from build123d import *

# Parameters (mm, degrees)
F0_R     = 3
F1_DEPTH = 15
F2_W     = 7
F2_H     = 5
F3_DEPTH = 10
F4_F1_R  = 2
F4_F2_R  = 2
F5_R     = 2


with BuildPart() as f1:
    # F0 (on Top) → F1 (new body)
    with BuildSketch(Plane.XY):
        with BuildLine():
            Line((-40.4142135624, -39), (-4.8904069139, -3.4761933515))
            ThreePointArc((-4.8904069139, -3.4761933515), (5.9789831367, -0.5017575617), (-4.2426406871, 4.2426406871))
            Line((-4.2426406871, 4.2426406871), (-42.4852813742, -34))
            Line((-42.4852813742, -34), (-104.8479702921, -34))
            Line((-104.8479702921, -34), (-87.5274622164, -44))
            Line((-87.5274622164, -44), (-90.4142135624, -39))
            Line((-90.4142135624, -39), (-40.4142135624, -39))
        make_face()
        Circle(F0_R, mode=Mode.SUBTRACT)
    extrude(amount=F1_DEPTH)

    # F2 (on face) → F3 (join)
    with BuildSketch(Plane(origin=(-4.2426406871, 4.2426406871, 0), x_dir=(-0.7071067812, -0.7071067812, 0), z_dir=(-0.7071067812, 0.7071067812, 0))):
        with Locations((36.5832611207, 7.5)):
            Rectangle(F2_W, F2_H)
    extrude(amount=F3_DEPTH)

    # F4: fillet of radius 2 on 9 edges, made by hand

    # F4_f1
    f4_f1_edges = [f1.edges().sort_by_distance(p)[0] for p in [
        (-36.1213203436, -20.5649711575, 10),
        (-36.1213203436, -20.5649711575, 5),
        (-31.1715728753, -15.6152236891, 5),
        (-31.1715728753, -15.6152236891, 10),
        (-37.1819805153, -14.5545635174, 10),
        (-37.1819805153, -14.5545635174, 5),
        (-34.7071067812, -12.0796897832, 7.5),
        (-39.6568542495, -17.0294372515, 7.5),
    ]]
    fillet(f4_f1_edges, radius=F4_F1_R)

    # F4_f2
    f4_f2_edges = [f1.edges().sort_by_distance(p)[0] for p in [
        (-32.5857864376, -24.1005050634, 7.5),
        (-32.1715728753, -23.686291501, 5.5857864376),
        (-32.1715728753, -23.686291501, 9.4142135624),
    ]]
    fillet(f4_f2_edges, radius=F4_F2_R)

    # F5
    f5_edges = [f1.edges().sort_by_distance(p)[0] for p in [
        (-104.84797, -34, 7.5),
        (-40.414214, -39, 7.5),
        (-42.485281, -34, 7.5),
    ]]
    fillet(f5_edges, radius=F5_R)


solid = f1.part
Design review of the part built by this model. Coordinates are the model's own, in mm. A direction names the side the tool comes from. Coordinates: 2 decimals unless noted, no trailing zeros. Loops run counter-clockwise (first coordinate to the right, second up) from the corner with the lowest first, then second, coordinate; pieces in that order, holes last. Notation, with made-up numbers: (-32.75, 82) -> (15.25, 82) arc R10 cw to (15.25, 93) -> close; hole circle Ø8 at (35.5, -27.5). An arc over 180 degrees is marked (long way). Use a Markdown table: item, result. Add a question column.
Item 1: We need section D-D, the plane x = -71. Write out the cut boundary in (y, z).
Item 2: Clearance check with flat-ended pins moving along their axes: P1, Ø2, axis at y = -38, z = 3.5, coming from the +X side; P2, Ø4.5, axis at x = -69.5, z = 7, coming from the -Y side; P3, Ø6, axis at x = -23.5, z = 7, coming from the +Y side. State where each tip first meets the part, or that it passes through.
Item 3: We need section C-C, the plane y = 0. Write out the cut boundary in (x, z).
Item 4: We need section A-A, the plane z = 13.5. Write out the cut boundary in (x, y), and give its area (3 significant figures).
Item 5: The part is to be moulded in two halves that separate along X. For faces 4 (the cylindrical face through (-31.605, -15.989, 5.601)), 5 (the cylindrical face through (-99.306, -35.447, 7.605)), 6 (the flat face through (-70, -34, 7)), say which applies: +X half, -X half, draft (parallel to the pull), parting line (faces both ways), or undercut.
Item 6: Machinability: for faces 1 (the cylindrical face through (-35.726, -20.11, 9.43)), 2 (the flat face through (-31.142, -15.645, 7.493)), 3 (the flat face through (-88.95, -41.54, 7.4)), which of the approach directions +Z, -Z, +X, -X, +Y, -Y give a long, thin tool a straight path to every point of the face, cutting with its end or side? Answer none if there is none.
Item 7: We need section B-B, the plane x = 0. Write out the cut boundary in (y, z), and give its area (3 significant figures).
Item 8: Wall thickness on L1, parallel to Y at x = 0, z = 5.5; L2, parallel to X at y = -17, z = 5.75; L3, parallel to Y at x = -68, z = 1.5: over which ranges is each line inside the solid? List them lowest first. Write a range as from..to.
Numbers:
| question | item | result |
|---|---|---|
| 1 | outline | (-39, 0) -> (-34, 0) -> (-34, 15) -> (-39, 15) -> close |
| 2 | P1 | stops at x = -38.41 |
| 2 | P2 | stops at y = -39 |
| 2 | P3 | stops at y = -12.01 |
| 3 | outline | (-8.49, 0) -> (-3, 0) -> (-3, 15) -> (-8.49, 15) -> close; (3, 0) -> (6, 0) -> (6, 15) -> (3, 15) -> close |
| 4 | outline | (-98.38, -37.73) -> (-87.53, -44) -> (-90.41, -39) -> (-41.24, -39) arc R2 ccw to (-39.83, -38.41) -> (-4.89, -3.48) arc R6 ccw (long way) to (-4.24, 4.24) -> (-41.9, -33.41) arc R2 cw to (-43.31, -34) -> (-97.38, -34) arc R2 ccw to start; hole circle Ø6 at (0, 0) |
| 4 | area | 638 mm^2 |
| 5 | face 4 | undercut |
| 5 | face 5 | -X half |
| 5 | face 6 | draft |
| 6 | face 1 | +Z, -X |
| 6 | face 2 | +Z, -Z, +Y |
| 6 | face 3 | +Z, -Z, +X |
| 7 | outline | (-6, 0) -> (-3, 0) -> (-3, 15) -> (-6, 15) -> close; (3, 0) -> (6, 0) -> (6, 15) -> (3, 15) -> close |
| 7 | area | 90.0 mm^2 |
| 8 | L1 | y = -6..-3, 3..6 |
| 8 | L2 | x = -38.39..-30.41, -25.49..-18.41 |
| 8 | L3 | y = -39..-34 |
